```python
from build123d import *

# Parameters (mm, degrees)
EXTRUSION1_DEPTH = 182
CONG_1_R         = 0.5


with BuildPart() as part:
    # Esquisse1 → Extrusion1 (new body)
    with BuildSketch(Plane(origin=(0, 0, 0), x_dir=(1, 0, 0), z_dir=(0, 1, 0))):
        with BuildLine():
            Line((7.5, 0), (-7.5, 0))
            Line((-7.5, 0), (-7.5, 4))
            ThreePointArc((-7.5, 4), (-8.5, 5.75), (-7.5, 7.5))
            Line((-7.5, 7.5), (-6.9, 7.5))
            Line((-6.9, 7.5), (-6.9, 7.114734406))
            ThreePointArc((-6.9, 7.114734406), (-7.9, 5.75), (-6.9, 4.385265594))
            Line((-6.9, 4.385265594), (-6.9, 0.6))
            Line((-6.9, 0.6), (6.9, 0.6))
            Line((6.9, 0.6), (6.9, 4.385265594))
            ThreePointArc((6.9, 4.385265594), (7.9, 5.75), (6.9, 7.114734406))
            Line((6.9, 7.114734406), (6.9, 7.5))
            Line((6.9, 7.5), (7.5, 7.5))
            ThreePointArc((7.5, 7.5), (8.5, 5.75), (7.5, 4))
            Line((7.5, 4), (7.5, 0))
        make_face()
    extrude(amount=EXTRUSION1_DEPTH)

    # Congé1
    cong_1_edges = [part.edges().sort_by_distance(p)[0] for p in [
        (7.5, 91, 0),
        (-7.5, 91, 0),
    ]]
    fillet(cong_1_edges, radius=CONG_1_R)


solid = part.part
```
Read the model definition and answer for the solid it produces. Units are mm, in the model's axes. A direction names the side the tool comes from. Give positions to 0.01 mm unless a question says otherwise; leave off trailing zeros. Write each loop counter-clockwise with the first axis right and the second up, starting at its lowest first coordinate (ties: lowest second). Pieces come first, ordered by that corner, then holes. Notation, with made-up numbers: (44, 37.5) - (66, 37.5) arc R34 ccw to (66, 75.5) - close; hole circle Ø10 at (81.5, -5). An arc over 180 degrees is marked (long way). Write item = value, one per line. Start each with the question number.
Item 1: Find section C-C (x = -4.5). Give the vertices of the cut face in (y, z), then the cut area to 3 significant figures.
Item 2: The mould has two halves that part along X. Classify faces 5 (the flat face through (0, 90, -0.6)), 6 (the cylindrical face through (-8.5, 89.7, -5.7)), 7 (the flat face through (0, 90, 0)): +X half, -X half, draft (parallel to the pull), parting line (faces both ways), or undercut.
Item 3: A tool of negligible diameter and unlimited length cuts with its end or side. For faces 1 (the flat face through (7.5, 90, -2)), 2 (the flat face through (-7.5, 90, -2)), 3 (the flat face through (-6.9, 90, -3)), 4 (the flat face through (1.3, 0, -0.4)), from which of +Z, -Z, +X, -X, +Y, -Y can it reach the whole face along a straight path? Write none if from no direction.
Item 4: Find section B-B (y = 12.5). Give the vertices of the cut face in (x, z).
Item 5: Each of these flat-tipped pins is pushed along its axis until it touches: P1, Ø3, axis at x = -6, y = 91.5, coming from the -Z side; P2, Ø3, axis at y = 73.5, z = -3, coming from the +X side; P3, Ø3, axis at y = 124.5, z = -2, coming from the -X side; P4, Ø8, axis at x = 2, y = 76.5, coming from the -Z side. Where does it stop, or does it pass through?
Item 6: Find section A-A (z = -2.75). Give the vertices of the cut face in (x, y), then the cut area to 3 significant figures.
Item 7: Find the intervals of material crossed by probe 1 along X at (y, z) = (152.5, -1.75); probe 2 along X at (y, z) = (86.5, -6); probe 3 along Z at (x, y) = (6.25, 116), in increasing order. Write a range as [from, to].
Response:
q1.outline = (0, -0.6) - (182, -0.6) - (182, 0) - (0, 0) - close
q1.area = 109 mm²
q2.face_5 = undercut
q2.face_6 = -X half
q2.face_7 = draft
q3.face_1 = +Z, +X, +Y, -Y
q3.face_2 = +Z, -X, +Y, -Y
q3.face_3 = -Z, +Y, -Y
q3.face_4 = +Z, -Z, +X, -X, -Y
q4.outline = (-7.5, -7.5) - (-6.9, -7.5) - (-6.9, -7.11) arc R1.43 cw to (-6.9, -4.39) - (-6.9, -0.6) - (6.9, -0.6) - (6.9, -4.39) arc R1.43 cw to (6.9, -7.11) - (6.9, -7.5) - (7.5, -7.5) arc R2.03 ccw to (7.5, -4) - (7.5, -0.5) arc R0.5 ccw to (7, 0) - (-7, 0) arc R0.5 ccw to (-7.5, -0.5) - (-7.5, -4) arc R2.03 ccw to start
q5.P1 = -7.5
q5.P2 = 8.07
q5.P3 = -7.5
q5.P4 = -0.6
q6.outline = (-7.5, 0) - (-6.9, 0) - (-6.9, 182) - (-7.5, 182) - close; (6.9, 0) - (7.5, 0) - (7.5, 182) - (6.9, 182) - close
q6.area = 218 mm²
q7.probe_1 = [-7.5, -6.9], [6.9, 7.5]
q7.probe_2 = [-8.48, -7.88], [7.88, 8.48]
q7.probe_3 = [-0.6, 0]
